```python
from build123d import *

# Parameters (mm, degrees)
SKETCH1_R               = 74.676
BOSS_EXTRUDE1_DEPTH     = 3.175
CUT_EXTRUDE1_REACH      = 107.656
SKETCH2_R               = 7
CUT_EXTRUDE3_DEPTH      = 106.655527906
CUT_EXTRUDE3_DEPTH_BACK = 106.655527906
SKETCH4_R               = 3.175
M4_CLEARANCE_HOLE1_D    = 4.5
CUT_EXTRUDE4_REACH      = 107.656
SKETCH8_R               = 1.89865
CUT_EXTRUDE5_REACH      = 107.656
SKETCH9_R               = 2.032


with BuildPart() as part:
    # Sketch1 → Boss-Extrude1 (new body)
    with BuildSketch(Plane(origin=(0, 0, 0), x_dir=(1, 0, 0), z_dir=(0, 1, 0))):
        with Locations(Location((0, 0, 0), (0, 0, 270))):
            Circle(SKETCH1_R)
    extrude(amount=BOSS_EXTRUDE1_DEPTH)

    # Sketch2 → Cut-Extrude1 (cut, up to next)
    with BuildSketch(Plane(origin=(0, 3.175, 0), x_dir=(1, 0, 0), z_dir=(0, 1, 0)), mode=Mode.PRIVATE) as cut_extrude1_sk1:
        with Locations(Location((0, 0, 0), (0, 0, 270))):
            Circle(SKETCH2_R)
    cut_extrude1_tool1 = extrude(cut_extrude1_sk1.sketch, amount=-CUT_EXTRUDE1_REACH, mode=Mode.PRIVATE) & part.part
    add(cut_extrude1_tool1.solids().sort_by_distance((0, 3.175, 0))[0], mode=Mode.SUBTRACT)

    # Sketch4 → Cut-Extrude3 (cut, two sides: drawn at the far end of the back side and taken through both)
    with BuildSketch(Plane(origin=(0, 3.175, 0), x_dir=(1, 0, 0), z_dir=(0, 1, 0)).offset(-CUT_EXTRUDE3_DEPTH_BACK)):
        with Locations(Location((-22.225, 0, 0), (0, 0, 270))):
            Circle(SKETCH4_R)
        with Locations(Location((22.225, 0, 0), (0, 0, 270))):
            Circle(SKETCH4_R)
    extrude(amount=CUT_EXTRUDE3_DEPTH + CUT_EXTRUDE3_DEPTH_BACK, mode=Mode.SUBTRACT)

    # M4 Clearance Hole1 (through all)
    with Locations(Plane(origin=(0, 3.175, 0), x_dir=(1, 0, 0), z_dir=(0, 1, 0))):
        with Locations((-8, 8), (8, 8), (8, -8), (-8, -8)):
            Hole(M4_CLEARANCE_HOLE1_D / 2)

    # Sketch8 → Cut-Extrude4 (cut, up to next)
    with BuildSketch(Plane(origin=(0, 3.175, 0), x_dir=(1, 0, 0), z_dir=(0, 1, 0)), mode=Mode.PRIVATE) as cut_extrude4_sk1:
        with Locations(Location((19.05, 38.1, 0), (0, 0, 270))):
            Circle(SKETCH8_R)
    cut_extrude4_tool1 = extrude(cut_extrude4_sk1.sketch, amount=-CUT_EXTRUDE4_REACH, mode=Mode.PRIVATE) & part.part
    # Sketch8 → Cut-Extrude4 (cut, up to next)
    with BuildSketch(Plane(origin=(0, 3.175, 0), x_dir=(1, 0, 0), z_dir=(0, 1, 0)), mode=Mode.PRIVATE) as cut_extrude4_sk2:
        with Locations(Location((-19.05, 38.1, 0), (0, 0, 270))):
            Circle(SKETCH8_R)
    cut_extrude4_tool2 = extrude(cut_extrude4_sk2.sketch, amount=-CUT_EXTRUDE4_REACH, mode=Mode.PRIVATE) & part.part
    add(cut_extrude4_tool1.solids().sort_by_distance((19.05, 3.175, -38.1))[0], mode=Mode.SUBTRACT)
    add(cut_extrude4_tool2.solids().sort_by_distance((-19.05, 3.175, -38.1))[0], mode=Mode.SUBTRACT)

    # Sketch9 → Cut-Extrude5 (cut, up to next)
    with BuildSketch(Plane(origin=(0, 3.175, 0), x_dir=(1, 0, 0), z_dir=(0, 1, 0)), mode=Mode.PRIVATE) as cut_extrude5_sk1:
        with Locations(Location((-8, -22.86, 0), (0, 0, 270))):
            Circle(SKETCH9_R)
    cut_extrude5_tool1 = extrude(cut_extrude5_sk1.sketch, amount=-CUT_EXTRUDE5_REACH, mode=Mode.PRIVATE) & part.part
    # Sketch9 → Cut-Extrude5 (cut, up to next)
    with BuildSketch(Plane(origin=(0, 3.175, 0), x_dir=(1, 0, 0), z_dir=(0, 1, 0)), mode=Mode.PRIVATE) as cut_extrude5_sk2:
        with Locations(Location((-8, -66.04, 0), (0, 0, 270))):
            Circle(SKETCH9_R)
    cut_extrude5_tool2 = extrude(cut_extrude5_sk2.sketch, amount=-CUT_EXTRUDE5_REACH, mode=Mode.PRIVATE) & part.part
    add(cut_extrude5_tool1.solids().sort_by_distance((-8, 3.175, 22.86))[0], mode=Mode.SUBTRACT)
    add(cut_extrude5_tool2.solids().sort_by_distance((-8, 3.175, 66.04))[0], mode=Mode.SUBTRACT)


solid = part.part
```
Verification items for the finished model (mm, model axes). Round coordinates to 2 decimals unless told otherwise and drop trailing zeros. Write each loop counter-clockwise with the first axis right and the second up, starting at its lowest first coordinate (ties: lowest second). Pieces come first, ordered by that corner, then holes. Notation, with made-up numbers: (16, -34.75) -> (20, -34.75) arc R11 cw to (20, -15.75) -> close; hole circle Ø8 at (77, -40). An arc over 180 degrees is marked (long way). Write each question's results on one line, items separated by ' | '. Start each with the question number.
1. Material ranges on probe 1 along Z at (x, y) = (8, 1.45); probe 2 along Z at (x, y) = (-3, 1.35); probe 3 along Z at (x, y) = (-9.5, 2.25), recorded low to high. Write a range as from..to.
2. Cross-section at C-C (y = 1.6). Count the separate pieces of the cut face and the enclosed holes in it, then the cut area to 3 significant figures.
3. Cross-section at D-D (z = 66.04). Enter the section's corners in (x, y) (3 decimals), then the cut area to 3 significant figures.
4. Cross-section at A-A (x = 0). Enter the section's corners in (y, z) (3 decimals), then the cut area to 3 significant figures.
5. Depth check by flat-ended pin: P1, Ø3.5, axis at x = -8, z = 22.86, coming from the -Y side; P2, Ø5.5, axis at x = -8, z = 66.04, coming from the -Y side. Enter the tip coordinate at first touch or a pass-through.
6. Cross-section at B-B (z = 0). Enter the section's corners in (x, y) (3 decimals), then the cut area to 3 significant figures.
7. Draft check along Z on faces 1 (the cylindrical face through (22.431, 1.565, 71.228)), 2 (the cylindrical face through (-17.45, 1.61, -37.08)), 3 (the flat face through (-16, 3.175, -1)). Enter one of: +Z half, -Z half, draft (parallel to the pull), parting line (faces both ways), or undercut.
Solutions:
1) probe 1: z = -74.25..-10.25, -5.75..5.75, 10.25..74.25 | probe 2: z = -74.62..-6.32, 6.32..74.62 | probe 3: z = -74.07..-9.68, -6.32..6.32, 9.68..21.49, 24.23..64.67, 67.41..74.07
2) separate pieces: 1 | enclosed holes: 11 | area: 17,200 mm2
3) outline: (-34.86, 0) -> (-10.032, 0) -> (-10.032, 3.175) -> (-34.86, 3.175) -> close; (-5.968, 0) -> (34.86, 0) -> (34.86, 3.175) -> (-5.968, 3.175) -> close | area: 208 mm2
4) outline: (0, -74.676) -> (3.175, -74.676) -> (3.175, -7) -> (0, -7) -> close; (0, 7) -> (3.175, 7) -> (3.175, 74.676) -> (0, 74.676) -> close | area: 430 mm2
5) P1: passes through | P2: stops at y = 0
6) outline: (-74.676, 0) -> (-25.4, 0) -> (-25.4, 3.175) -> (-74.676, 3.175) -> close; (-19.05, 0) -> (-7, 0) -> (-7, 3.175) -> (-19.05, 3.175) -> close; (7, 0) -> (19.05, 0) -> (19.05, 3.175) -> (7, 3.175) -> close; (25.4, 0) -> (74.676, 0) -> (74.676, 3.175) -> (25.4, 3.175) -> close | area: 389 mm2
7) face 1: parting line | face 2: undercut | face 3: draft
